Autodesk Inventor part; units mm, degrees
ref_plane "YZ Plane" through (0, 0, 0) normal (1, 0, 0) x (0, 1, 0)
ref_plane "XZ Plane" through (0, 0, 0) normal (0, 1, 0) x (-1, 0, 0)
ref_plane "XY Plane" through (0, 0, 0) normal (0, 0, 1) x (1, 0, 0)
sketch "Sketch1" plane through (0, 0, 0) normal (0, 1, 0) x (-1, 0, 0)
  line L0 (-10, 10) -> (10, 10)
  line L1 (10, 10) -> (10, -10)
  line L2 (10, -10) -> (-10, -10)
  line L3 (-10, -10) -> (-10, 10)
  line L4 (-10, 10) -> (10, -10) construction
  line L5 (10, 10) -> (-10, -10) construction
  point P0 (0, 0)
  dimension "d0" = 20
  dimension "d1" = 20
extrude "Extrusion1" add sketch "Sketch1" along normal blind 0.5
sketch "Sketch2" plane through (0, 0.5, 0) normal (0, 1, 0) x (1, 0, 0)
  line L0 (10, 10) -> (-10, 10)
  line L1 (-10, 10) -> (-10, -10)
  line L2 (-10, -10) -> (10, -10)
  line L3 (10, -10) -> (10, 10)
  line L4 (-10, -10) -> (10, -10)
  line L5 (10, -10) -> (-10, -10)
  line L6 (-10, -10) -> (-10, -10.5)
  line L7 (-10, -10.5) -> (10, -10.5)
  line L8 (10, -10.5) -> (10, -10)
  point P0 (0, 0)
  dimension "d4" = 0.5
extrude "Extrusion2" add sketch "Sketch2" along normal blind 20 contours L8 L7 L6 L2
sketch "Sketch3" plane through (10, 0.5, 10.5) normal (1, 0, 0) x (0, 0, -1)
  line L0 (0.5, 0) -> (20.5, 0)
  line L1 (0.5, -0.5) -> (0.5, 0)
  circle A0 centre (0.5, 0) radius 0.5
  line L2 (0, 0) -> (0.5, 0)
  line L3 (0.5, 0) -> (0.5, 20)
  line L4 (0, 20) -> (0.5, 20)
  line L5 (0, 0) -> (0, 20)
  point P0 (10.5, -0.5)
extrude "Extrusion3" add sketch "Sketch3" against normal up to surface (20 mm away) contours L1 A0 L2
sketch "Sketch4" plane through (0, 0.5, 0) normal (0, 1, 0) x (1, 0, 0)
  point P0 (0, 0)
properties part number "l bracket" material "Stainless Steel"
Work out the finished part from the listing and answer in its coordinate system (mm). A direction names the side the tool comes from. Give positions to 0.01 mm unless a question says otherwise; leave off trailing zeros. Loops run counter-clockwise (first coordinate to the right, second up) from the corner with the lowest first, then second, coordinate; pieces in that order, holes last. Notation, with made-up numbers: (44.5, 44.25) -> (82.5, 44.25) arc R32 ccw to (82.5, 73.25) -> close; hole circle Ø11 at (29.5, -4.75). An arc over 180 degrees is marked (long way). Use a Markdown table: item, result. Add a question column.
1) The part is cut by section B-B, the plane y = 5.25. Determine the outline of the cut face in (x, z), plus the area to 3 significant figures.
2) Each of these flat-tipped pins is pushed along its axis until it touches: P1, Ø2, axis at x = 4.5, y = 5, coming from the -Z side; P2, Ø6, axis at x = -2, z = 2, coming from the +Y side; P3, Ø10, axis at y = 6.5, z = -6.5, coming from the -X side. Where does it stop, or does it pass through?
3) Consider line 1 along Z through (x, y) = (5, 5.5); line 2 along Y through (x, z) = (2.25, 8.25). Determine where each line is inside the solid, lowest interval first.
4) The part is cut by section C-C, the plane z = -6.75. Determine the outline of the cut face in (x, y).
5) Which of the six approach directions +Z, -Z, +X, -X, +Y, -Y give full straight-line access (tool end or side, diameter ignored) to faces 1 (the flat face through (0, 0.5, 0)), 2 (the flat face through (0, 0, 0))?
6) The part is cut by section A-A, the plane x = 3.25. Determine the outline of the cut face in (y, z), plus the area to 3 significant figures.
Reported:
| question | item | result |
|---|---|---|
| 1 | outline | (-10, 10) -> (10, 10) -> (10, 10.5) -> (-10, 10.5) -> close |
| 1 | area | 10.0 mm^2 |
| 2 | P1 | stops at z = 10 |
| 2 | P2 | stops at y = 0.5 |
| 2 | P3 | passes through |
| 3 | line 1 | z = 10 to 10.5 |
| 3 | line 2 | y = 0 to 0.5 |
| 4 | outline | (-10, 0) -> (10, 0) -> (10, 0.5) -> (-10, 0.5) -> close |
| 5 | face 1 | -Z, +X, -X, +Y |
| 5 | face 2 | +Z, -Z, +X, -X, -Y |
| 6 | outline | (0, -10) -> (0.5, -10) -> (0.5, 10) -> (20.5, 10) -> (20.5, 10.5) -> (0.5, 10.5) arc R0.5 ccw to (0, 10) -> close |
| 6 | area | 20.2 mm^2 |
